Part print with two shaded views. Sizes in mm from the minimum x, y, z corner. A direction names the side the tool comes from. Give positions to 0.01 mm unless a question says otherwise; leave off trailing zeros. Write each loop counter-clockwise with the first axis right and the second up, starting at its lowest first coordinate (ties: lowest second). Pieces come first, ordered by that corner, then holes.
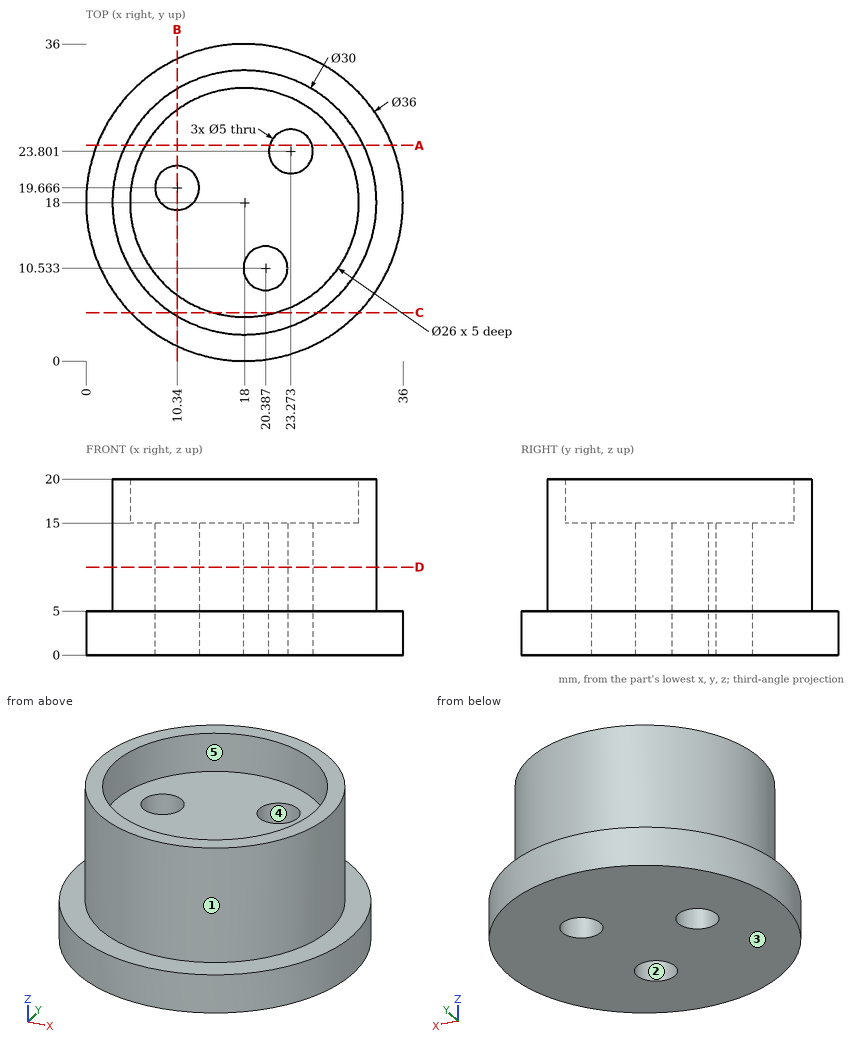
1) Mould opens along Y. For the marked faces 1, 2 and 3 say: +Y half, -Y half, draft (parallel to the pull), parting line (faces both ways), or undercut.
Check result:
face 1: parting line
face 2: undercut
face 3: draft
2) Saw through at C-C (y = 5.5). Write the cut outline in (x, z).
Check result:
outline: (5.05, 0) - (30.95, 0) - (30.95, 5) - (26.29, 5) - (26.29, 20) - (21.57, 20) - (21.57, 15) - (14.43, 15) - (14.43, 20) - (9.71, 20) - (9.71, 5) - (5.05, 5) - close
3) 3-axis set-ups, long thin cutter, end or side, ignore diameter. For the marked faces 4 and 5: which of +Z, -Z, +X, -X, +Y, -Y reach the whole face in a straight line?
Check result:
face 4: +Z, -Z
face 5: +Z
4) Saw through at D-D (z = 10). Write the cut outline in (x, y), and give its area (3 significant figures).
Check result:
outline: circle Ø30 at (18, 18); hole circle Ø5 at (10.34, 19.67); hole circle Ø5 at (20.39, 10.53); hole circle Ø5 at (23.27, 23.8)
area: 648 mm2
5) Saw through at A-A (y = 24.5). Write the cut outline in (x, z) (1 decimal), and give its area (3 significant figures).
Check result:
outline: (1.2, 0) - (20.9, 0) - (20.9, 15) - (6.7, 15) - (6.7, 20) - (4.5, 20) - (4.5, 5) - (1.2, 5) - close; (25.7, 0) - (34.8, 0) - (34.8, 5) - (31.5, 5) - (31.5, 20) - (29.3, 20) - (29.3, 15) - (25.7, 15) - close
area: 389 mm2
6) Saw through at B-B (x = 10.34). Write the cut outline in (y, z), and give its area (3 significant figures).
Check result:
outline: (1.71, 0) - (17.17, 0) - (17.17, 15) - (7.5, 15) - (7.5, 20) - (5.1, 20) - (5.1, 5) - (1.71, 5) - close; (22.17, 0) - (34.29, 0) - (34.29, 5) - (30.9, 5) - (30.9, 20) - (28.5, 20) - (28.5, 15) - (22.17, 15) - close
area: 370 mm2
7) Flat gauge pins, fed straight in: P1, Ø1, axis at y = 19.5, z = 14, coming from the +X side; P2, Ø4.5, axis at x = 10.34, y = 19.67, coming from the +Z side; P3, Ø1.5, axis at x = 21, y = 29.5, coming from the +Z side; P4, Ø18, axis at x = 11, y = 11, coming from the +Z side. Where does each tip first touch, or does it go through?
Check result:
P1: stops at x = 32.97
P2: passes through
P3: stops at z = 15
P4: stops at z = 20
8) Drill centre lines: L1, parallel to Z at x = 17, y = 16.5; L2, parallel to Z at x = 4, y = 7; L3, parallel to Y at x = 25, z = 16.75 (1 decimal). Where is each one in solid material? Low to high.
Check result:
L1: z = 0 to 15
L2: z = 0 to 5
L3: y = 4.7 to 7, 29 to 31.3
